from build123d import *

# Parameters (mm, degrees)
SKETCH_1_R         = 2.1
EXTRUDE_1_DEPTH    = 75
VERRUNDUNG1_R      = 1
SKETCH1_R          = 3
CUT_EXTRUDE1_DEPTH = 41


with BuildPart() as part:
    # 草图1 → 凸台-拉伸1 (new body)
    with BuildSketch(Plane.XY):
        Polygon((5.71, 20), (-5.71, 20), (-6.9, 18.81), (-6.9, 18.2), (-4.5, 18.2), (-4.5, 16.489949494), (-7.089949494, 13.9), (-12.910050506, 13.9), (-15.5, 16.489949494), (-15.5, 18.2), (-13.1, 18.2), (-13.1, 18.81), (-14.29, 20), (-20, 20), (-20, 14.29), (-18.81, 13.1), (-18.2, 13.1), (-18.2, 15.5), (-16.489949494, 15.5), (-13.9, 12.910050506), (-13.9, 7.089949494), (-16.489949494, 4.5), (-18.2, 4.5), (-18.2, 6.9), (-18.81, 6.9), (-20, 5.71), (-20, -5.71), (-18.81, -6.9), (-18.2, -6.9), (-18.2, -4.5), (-16.489949494, -4.5), (-13.9, -7.089949494), (-13.9, -12.910050506), (-16.489949494, -15.5), (-18.2, -15.5), (-18.2, -13.1), (-18.81, -13.1), (-20, -14.29), (-20, -20), (-14.29, -20), (-13.1, -18.81), (-13.1, -18.2), (-15.5, -18.2), (-15.5, -16.489949494), (-12.910050506, -13.9), (-7.089949494, -13.9), (-4.5, -16.489949494), (-4.5, -18.2), (-6.9, -18.2), (-6.9, -18.81), (-5.71, -20), (5.71, -20), (6.9, -18.81), (6.9, -18.2), (4.5, -18.2), (4.5, -16.489949494), (7.089949494, -13.9), (12.910050506, -13.9), (15.5, -16.489949494), (15.5, -18.2), (13.1, -18.2), (13.1, -18.81), (14.29, -20), (20, -20), (20, -14.29), (18.81, -13.1), (18.2, -13.1), (18.2, -15.5), (16.489949494, -15.5), (13.9, -12.910050506), (13.9, -7.089949494), (16.489949494, -4.5), (18.2, -4.5), (18.2, -6.9), (18.81, -6.9), (20, -5.71), (20, 5.71), (18.81, 6.9), (18.2, 6.9), (18.2, 4.5), (16.489949494, 4.5), (13.9, 7.089949494), (13.9, 12.910050506), (16.489949494, 15.5), (18.2, 15.5), (18.2, 13.1), (18.81, 13.1), (20, 14.29), (20, 20), (14.29, 20), (13.1, 18.81), (13.1, 18.2), (15.5, 18.2), (15.5, 16.489949494), (12.910050506, 13.9), (7.089949494, 13.9), (4.5, 16.489949494), (4.5, 18.2), (6.9, 18.2), (6.9, 18.81), align=None)
        with Locations((-10, 10)):
            Circle(SKETCH_1_R, mode=Mode.SUBTRACT)
        with Locations((-10, -10)):
            Circle(SKETCH_1_R, mode=Mode.SUBTRACT)
        with Locations((10, -10)):
            Circle(SKETCH_1_R, mode=Mode.SUBTRACT)
        with Locations((10, 10)):
            Circle(SKETCH_1_R, mode=Mode.SUBTRACT)
        Polygon((-6.1, 6.1), (-6.1, 12.910050506), (-3, 16.010050506), (-3, 18.2), (3, 18.2), (3, 16.010050506), (6.1, 12.910050506), (6.1, 6.1), (12.910050506, 6.1), (16.010050506, 3), (18.2, 3), (18.2, -3), (16.010050506, -3), (12.910050506, -6.1), (6.1, -6.1), (6.1, -12.910050506), (3, -16.010050506), (3, -18.2), (-3, -18.2), (-3, -16.010050506), (-6.1, -12.910050506), (-6.1, -6.1), (-12.910050506, -6.1), (-16.010050506, -3), (-18.2, -3), (-18.2, 3), (-16.010050506, 3), (-12.910050506, 6.1), align=None, mode=Mode.SUBTRACT)
    extrude(amount=EXTRUDE_1_DEPTH)

    # Verrundung1
    verrundung1_edges = [part.edges().sort_by_distance(p)[0] for p in [
        (20, 20, 37.5),
        (20, -20, 37.5),
        (-20, -20, 37.5),
        (-20, 20, 37.5),
    ]]
    fillet(verrundung1_edges, radius=VERRUNDUNG1_R)

    # Sketch1 → Cut-Extrude1 (cut, through all)
    with BuildSketch(Plane.ZY.offset(20)):
        with Locations((41, 0)):
            Circle(SKETCH1_R)
    cut_extrude1 = extrude(amount=-CUT_EXTRUDE1_DEPTH, mode=Mode.SUBTRACT)

    # Mirror1: Cut-Extrude1 across plane
    add(cut_extrude1.mirror(Plane(origin=(0, 0, 0), x_dir=(0, 0, 1), z_dir=(-0.707106781, -0.707106781, 0))), mode=Mode.SUBTRACT)


solid = part.part
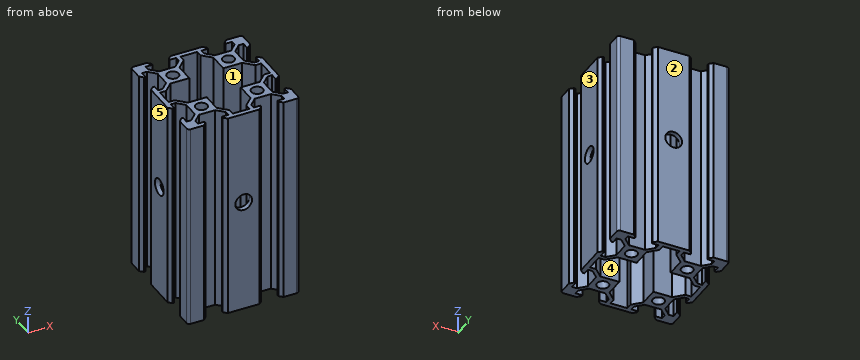
Geometry check sheet. Reference: the model listing, model coordinates, mm. Face numbers are marked on the shaded views. A direction names the side the tool comes from. Coordinates: 2 decimals unless noted, no trailing zeros. Loops run counter-clockwise (first coordinate to the right, second up) from the corner with the lowest first, then second, coordinate; pieces in that order, holes last. Notation, with made-up numbers: (-34.5, 45) - (-5.5, 45) arc R25 cw to (-5.5, 57) - close; hole circle Ø5 at (33, -36). An arc over 180 degrees is marked (long way). Use one line per item in the form item = value. Start each with the question number.
Item 1: Section check B-B, the plane y = -10. Enter the section's corners in (x, z).
Item 2: Section check A-A, the plane x = 0. Enter the section's corners in (y, z), and give its area (3 significant figures).
Item 3: Mould release check, pull along X, two halves, no side actions. Record for the marked faces 3, 4 and 5: +X half, -X half, draft (parallel to the pull), parting line (faces both ways), or undercut.
Item 4: Tool access check on the marked faces 1 and 2. Record the directions out of +Z, -Z, +X, -X, +Y, -Y that give a thin tool (end or side, any length) a straight path to the whole face; none if there is none.
Item 5: Section check C-C, the plane z = 5. Give the number of separate pieces and of enclosed holes in the cut face, and give its area (3 significant figures).
Item 6: Thickness scan on probe 1 along Y at (x, z) = (10, 18); probe 2 along X at (y, z) = (-18, 4.5). Record the ranges inside material, lowest first.
Item 7: Gauge pin test, flat ends, axial feed: pin 1 (4.5 mm diameter, centred on y = -11, z = 32, fed in from -X); pin 2 (5.5 mm diameter, centred on x = -10, z = 40, fed in from +Y); pin 3 (1.5 mm diameter, centred on y = -13.5, z = 43.5, fed in from -X). Record the tip position at first contact, or that the pin passes through.
Computed:
q1.outline = (-13.9, 0) - (-12.1, 0) - (-12.1, 75) - (-13.9, 75) - close; (-7.9, 0) - (-6.1, 0) - (-6.1, 75) - (-7.9, 75) - close; (6.1, 0) - (7.9, 0) - (7.9, 75) - (6.1, 75) - close; (12.1, 0) - (13.9, 0) - (13.9, 75) - (12.1, 75) - close
q2.outline = (-20, 0) - (-18.2, 0) - (-18.2, 38) - (-20, 38) - close; (-20, 44) - (-18.2, 44) - (-18.2, 75) - (-20, 75) - close; (18.2, 0) - (20, 0) - (20, 38) - (18.2, 38) - close; (18.2, 44) - (20, 44) - (20, 75) - (18.2, 75) - close
q2.area = 248 mm2
q3.face_3 = +X half
q3.face_4 = undercut
q3.face_5 = -X half
q4.face_1 = +Z, -Z
q4.face_2 = +Z, -Z, +X, -X, +Y
q5.separate_pieces = 1
q5.enclosed_holes = 5
q5.area = 472 mm2
q6.probe_1 = -13.9 to -12.1, -7.9 to -6.1, 6.1 to 7.9, 12.1 to 13.9
q6.probe_2 = -20 to -15.5, -4.5 to -3, 3 to 4.5, 15.5 to 20
q7.pin_1 = -18.96
q7.pin_2 = 13.9
q7.pin_3 = -19.96
